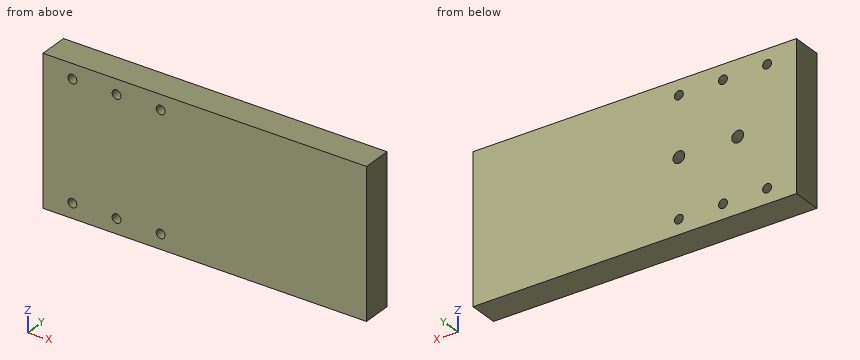
```python
from build123d import *

# Parameters (mm, degrees)
SKETCH_1_W          = 220
SKETCH_1_H          = 100
EXTRUDE_1_DEPTH     = 20
SKETCH_2_R          = 4
CUT_EXTRUDE_1_DEPTH = 10
SKETCH_3_R          = 3
CUT_EXTRUDE_2_DEPTH = 20


with BuildPart() as part:
    # Эскиз1 → Бобышка-Вытянуть1 (new body)
    with BuildSketch(Plane(origin=(0, 0, 0), x_dir=(1, 0, 0), z_dir=(0, 1, 0))):
        with Locations((110, 50)):
            Rectangle(SKETCH_1_W, SKETCH_1_H)
    extrude(amount=EXTRUDE_1_DEPTH)

    # Эскиз2 → Вырез-Вытянуть1 (cut)
    with BuildSketch(Plane(origin=(0, 20, 0), x_dir=(1, 0, 0), z_dir=(0, 1, 0))):
        with Locations(Location((80, 50, 0), (0, 0, 270))):
            Circle(SKETCH_2_R)
        with Locations(Location((40, 50, 0), (0, 0, 270))):
            Circle(SKETCH_2_R)
    extrude(amount=-CUT_EXTRUDE_1_DEPTH, mode=Mode.SUBTRACT)

    # Эскиз3 → Вырез-Вытянуть2 (cut)
    with BuildSketch(Plane(origin=(0, 20, 0), x_dir=(1, 0, 0), z_dir=(0, 1, 0))):
        with Locations(Location((20, 90, 0), (0, 0, 270))):
            Circle(SKETCH_3_R)
        with Locations(Location((50, 90, 0), (0, 0, 270))):
            Circle(SKETCH_3_R)
        with Locations(Location((80, 90, 0), (0, 0, 270))):
            Circle(SKETCH_3_R)
        with Locations(Location((20, 10, 0), (0, 0, 270))):
            Circle(SKETCH_3_R)
        with Locations(Location((50, 10, 0), (0, 0, 270))):
            Circle(SKETCH_3_R)
        with Locations(Location((80, 10, 0), (0, 0, 270))):
            Circle(SKETCH_3_R)
    extrude(amount=-CUT_EXTRUDE_2_DEPTH, mode=Mode.SUBTRACT)


solid = part.part
```
Geometry: final body of the model. Coordinates: model frame, mm. Coordinates: 2 decimals unless noted, no trailing zeros. Order: outer loops, then holes, each group sorted by start corner. A loop starts at its lowest first (then second) coordinate and runs counter-clockwise, first axis right, second up. Notation, with made-up numbers: M 77,63 L 85,63 A21 cw 85,77 Z; hole C 20,75 d2. An arc over 180 degrees is marked long. Answer as CSV lines item,"result".
Q1. First-contact query: P1, Ø4, axis at x = 40, z = -50, coming from the +Y side; P2, Ø3.5, axis at x = 80, z = -90, coming from the +Y side. Flat tips, straight axial feed; report the tip coordinate or a pass-through.
Answers:
P1,"stops at y = 10"
P2,"passes through"
Q2. Section C-C on z = -50. Return the cut outline in (x, y).
Answers:
outline,"M 0,0 L 220,0 L 220,20 L 84,20 L 84,10 L 76,10 L 76,20 L 44,20 L 44,10 L 36,10 L 36,20 L 0,20 Z"
Q3. Section B-B on x = 50. Return the cut outline in (y, z).
Answers:
outline,"M 0,-100 L 20,-100 L 20,-93 L 0,-93 Z; M 0,-87 L 20,-87 L 20,-13 L 0,-13 Z; M 0,-7 L 20,-7 L 20,0 L 0,0 Z"
Q4. Section D-D on x = 80. Return the cut outline in (y, z).
Answers:
outline,"M 0,-100 L 20,-100 L 20,-93 L 0,-93 Z; M 0,-87 L 20,-87 L 20,-54 L 10,-54 L 10,-46 L 20,-46 L 20,-13 L 0,-13 Z; M 0,-7 L 20,-7 L 20,0 L 0,0 Z"
Q5. Line query: probe 1 along X at (y, z) = (14, -10); probe 2 along X at (y, z) = (15.5, -50); probe 3 along X at (y, z) = (17, -47). Output: solid intervals per line, ascending. Write a range as [from, to].
Answers:
probe 1,"x = [0, 17], [23, 47], [53, 77], [83, 220]"
probe 2,"x = [0, 36], [44, 76], [84, 220]"
probe 3,"x = [0, 37.35], [42.65, 77.35], [82.65, 220]"
Q6. Section A-A on z = -10. Return the cut outline in (x, y), and give its area (3 significant figures).
Answers:
outline,"M 0,0 L 17,0 L 17,20 L 0,20 Z; M 23,0 L 47,0 L 47,20 L 23,20 Z; M 53,0 L 77,0 L 77,20 L 53,20 Z; M 83,0 L 220,0 L 220,20 L 83,20 Z"
area,"4,040 mm^2"
